Geometry check sheet. Reference: the model listing, model coordinates, mm. Face numbers are marked on the shaded views. A direction names the side the tool comes from. Round coordinates to 2 decimals unless told otherwise and drop trailing zeros. Order: outer loops, then holes, each group sorted by start corner. A loop starts at its lowest first (then second) coordinate and runs counter-clockwise, first axis right, second up. Notation, with made-up numbers: (24.25, 87.25) -> (43.25, 87.25) arc R32 cw to (43.25, 125.25) -> close; hole circle Ø8 at (80.25, -38). An arc over 180 degrees is marked (long way). Use a Markdown table: item, result. Add a question column.
Item 1: Material ranges on probe 1 along Z at (x, y) = (13.5, -4.25); probe 2 along Y at (x, z) = (7, 1), recorded low to high. Write a range as [from, to].
Item 2: Sectioned sample at C-C, the plane y = 3.5. Record the cut outline in (x, z) (3 decimals).
Item 3: Set-up check for the marked faces 1 and 2: record each of +Z, -Z, +X, -X, +Y, -Y from which the full face is reachable in a straight line by a thin tool's end or side.
Item 4: Sectioned sample at A-A, the plane y = 0. Record the cut outline in (x, z) (3 decimals).
Item 5: Sectioned sample at D-D, the plane z = 13.75. Record the cut outline in (x, y), and give its area (3 significant figures).
Item 6: Sectioned sample at B-B, the plane x = 11. Record the cut outline in (y, z).
Item 7: Gauge pin test, flat ends, axial feed: pin 1 Ø10 at (x, y) = (4, -3) entering from -Z; pin 2 Ø4 at (y, z) = (5, 10) entering from +X; pin 3 Ø8.5 at (x, y) = (12, -4) entering from +Z. Record the tip position at first contact, or that the pin passes through.
from build123d import *

# Parameters (mm, degrees)
EXTRUDE_THIN1_START = -11.1125
EXTRUDE_THIN1_DEPTH = 22.225
SKETCH4_R           = 2.0828
EXTRUDE3_DEPTH      = 27.127838741
CUT_EXTRUDE1_DEPTH  = 28.173622895


# Read off the part's stored shape, not the designer's step: Extrude-Thin1
with BuildPart() as part:
    # Extrude-Thin1 outline → Extrude-Thin1 (new body)
    with BuildSketch(Plane(origin=(0, 0, 0), x_dir=(1, 0, 0), z_dir=(0, 1, 0)).offset(EXTRUDE_THIN1_START)):
        with BuildLine():
            Line((2.286, -1.524), (19.05, -1.524))
            Line((19.05, -1.524), (19.05, 0))
            Line((19.05, 0), (2.286, 0))
            ThreePointArc((2.286, 0), (0.669553898, -0.669553898), (0, -2.286))
            Line((0, -2.286), (0, -15.875))
            Line((0, -15.875), (1.524, -15.875))
            Line((1.524, -15.875), (1.524, -2.286))
            ThreePointArc((1.524, -2.286), (1.747184633, -1.747184633), (2.286, -1.524))
        make_face()
    extrude(amount=EXTRUDE_THIN1_DEPTH)

    # Sketch4 → Extrude3 (cut, through all)
    with BuildSketch(Plane(origin=(1.524, 0, 0), x_dir=(0, 0, -1), z_dir=(1, 0, 0))):
        with Locations((-7.875, 0)):
            Circle(SKETCH4_R)
    extrude(amount=-EXTRUDE3_DEPTH, mode=Mode.SUBTRACT)

    # Sketch6 → Cut-Extrude1 (cut, through all)
    with BuildSketch(Plane.XY):
        with BuildLine():
            Line((6.05, 2.0828), (14.05, 2.0828))
            ThreePointArc((14.05, 2.0828), (16.1328, 0), (14.05, -2.0828))
            Line((14.05, -2.0828), (6.05, -2.0828))
            ThreePointArc((6.05, -2.0828), (3.9672, 0), (6.05, 2.0828))
        make_face()
    extrude(amount=CUT_EXTRUDE1_DEPTH, mode=Mode.SUBTRACT)


solid = part.part
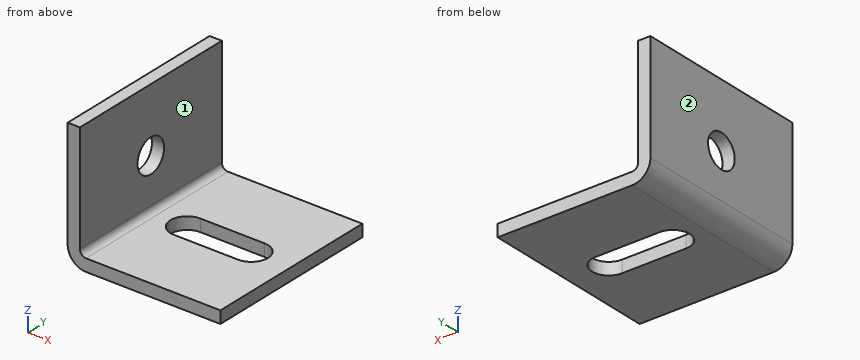
Found:
| question | item | result |
|---|---|---|
| 1 | probe 1 | z = [0, 1.52] |
| 1 | probe 2 | y = [-11.11, -2.08], [2.08, 11.11] |
| 2 | outline | (0, 2.286) arc R2.286 ccw to (2.286, 0) -> (19.05, 0) -> (19.05, 1.524) -> (2.286, 1.524) arc R0.762 cw to (1.524, 2.286) -> (1.524, 15.875) -> (0, 15.875) -> close |
| 3 | face 1 | +Z, +X, +Y, -Y |
| 3 | face 2 | +Z, -Z, -X, +Y, -Y |
| 4 | outline | (0, 2.286) arc R2.286 ccw to (2.286, 0) -> (3.967, 0) -> (3.967, 1.524) -> (2.286, 1.524) arc R0.762 cw to (1.524, 2.286) -> (1.524, 5.792) -> (0, 5.792) -> close; (0, 9.958) -> (1.524, 9.958) -> (1.524, 15.875) -> (0, 15.875) -> close; (16.133, 0) -> (19.05, 0) -> (19.05, 1.524) -> (16.133, 1.524) -> close |
| 5 | outline | (0, -11.11) -> (1.52, -11.11) -> (1.52, 11.11) -> (0, 11.11) -> close |
| 5 | area | 33.9 mm2 |
| 6 | outline | (-11.11, 0) -> (-2.08, 0) -> (-2.08, 1.52) -> (-11.11, 1.52) -> close; (2.08, 0) -> (11.11, 0) -> (11.11, 1.52) -> (2.08, 1.52) -> close |
| 7 | pin 1 | stops at z = 0 |
| 7 | pin 2 | stops at x = 1.52 |
| 7 | pin 3 | stops at z = 1.52 |
